Verification items for the finished model (mm, model axes). A direction names the side the tool comes from. Round coordinates to 2 decimals unless told otherwise and drop trailing zeros. Order: outer loops, then holes, each group sorted by start corner. A loop starts at its lowest first (then second) coordinate and runs counter-clockwise, first axis right, second up. Notation, with made-up numbers: M -17,68 L 33,68 A30 cw 33,107 Z; hole C 56.5,75 d5. An arc over 180 degrees is marked long. Answer as a JSON object with one key per item and string values. Group by question number.
```python
from build123d import *

# Parameters (mm, degrees)
IZIM1_R                                           = 52.5
IZIM1_R_2                                         = 21
Y_KSEKLIK_EKSTR_ZYON1_DEPTH                       = 10
Y_KSEKLIK_EKSTR_ZYON1_DRAFT                       = 4.33
M8_ALT_GEN_ALYAN_BA_L_K_R_VIDA_IN_HAV_D           = 9
M8_ALT_GEN_ALYAN_BA_L_K_R_VIDA_IN_HAV_DEPTH       = 22.25
M8_ALT_GEN_ALYAN_BA_L_K_R_VIDA_IN_HAV_CBORE_D     = 15
M8_ALT_GEN_ALYAN_BA_L_K_R_VIDA_IN_HAV_CBORE_DEPTH = 8.6
M8_ALT_GEN_ALYAN_BA_L_K_R_VIDA_IN_HAV_TIP         = 2.703872786
IZIM4_R                                           = 22
IZIM4_R_2                                         = 21
Y_KSEKLIK_EKSTR_ZYON2_DEPTH                       = 10


with BuildPart() as part:
    # Çizim1 → Yükseklik-Ekstrüzyon1 (with draft: the straight prism first)
    with BuildSketch(Plane.XY):
        Circle(IZIM1_R)
        Circle(IZIM1_R_2, mode=Mode.SUBTRACT)
    extrude(amount=Y_KSEKLIK_EKSTR_ZYON1_DEPTH)
    # Yükseklik-Ekstrüzyon1: the draft: its side faces are tilted about the plane it starts from
    y_kseklik_ekstr_zyon1_sides = [part.faces().sort_by_distance(p)[0] for p in [
        (-52.5, 0, 5),
        (-21, 0, 5),
    ]]
    draft(y_kseklik_ekstr_zyon1_sides, Plane.XY, Y_KSEKLIK_EKSTR_ZYON1_DRAFT)

    # M8 Altıgen Alyan Başlı Kör Vida İçin Havşa1
    with Locations(Plane.XY.offset(10)):
        with Locations((14.701198769, 35.58264682), (-35.58264682, 14.701198769), (-14.701198769, -35.58264682), (35.58264682, -14.701198769)):
            CounterBoreHole(M8_ALT_GEN_ALYAN_BA_L_K_R_VIDA_IN_HAV_D / 2, M8_ALT_GEN_ALYAN_BA_L_K_R_VIDA_IN_HAV_CBORE_D / 2, M8_ALT_GEN_ALYAN_BA_L_K_R_VIDA_IN_HAV_CBORE_DEPTH, depth=M8_ALT_GEN_ALYAN_BA_L_K_R_VIDA_IN_HAV_DEPTH)
            with Locations((0, 0, -(M8_ALT_GEN_ALYAN_BA_L_K_R_VIDA_IN_HAV_DEPTH + M8_ALT_GEN_ALYAN_BA_L_K_R_VIDA_IN_HAV_TIP / 2))):  # 118° drill point
                Cone(0, M8_ALT_GEN_ALYAN_BA_L_K_R_VIDA_IN_HAV_D / 2, M8_ALT_GEN_ALYAN_BA_L_K_R_VIDA_IN_HAV_TIP, mode=Mode.SUBTRACT)

    # Çizim4 → Yükseklik-Ekstrüzyon2 (add)
    with BuildSketch(Plane.XY):
        Circle(IZIM4_R)
        Circle(IZIM4_R_2, mode=Mode.SUBTRACT)
    extrude(amount=Y_KSEKLIK_EKSTR_ZYON2_DEPTH)


solid = part.part
```
Q1. Release check for a two-part mould opening along X. For faces 3 (the face through (22, 1, 10)), 4 (the face through (-39.875, 16.053, 0.69)), 5 (the face through (49.399, 15.556, 9.374)), 6 (the face through (-11, -39, 1.4)) record: released by +X, released by -X, zero draft, split by the parting line, or undercut.
Q2. Tool access check on faces 1 (the face through (-1, -23, 0)), 2 (the face through (-16.327, -42.904, 5.76)). Record the directions out of +Z, -Z, +X, -X, +Y, -Y that give a thin tool (end or side, any length) a straight path to the whole face; none if there is none.
Q3. Thickness scan on line 1 (X direction, y = 17, z = 5.5); line 2 (Y direction, x = 8.5, z = 8.75); line 3 (Y direction, x = 18, z = 1). Record the ranges inside material, lowest first. Write a range as from..to.
Q4. Cross-section at D-D, the plane z = 3. Record the cut outline in (x, y), then the cut area to 3 significant figures.
Q5. Gauge pin test, flat ends, axial feed: pin 1 Ø3 at (x, z) = (33.5, 3) entering from +Y; pin 2 Ø5 at (x, z) = (-38, 6.5) entering from +Y; pin 3 Ø4.5 at (x, y) = (38.5, -15) entering from +Z. Record the tip position at first contact, or that the pin passes through.
Q6. Cross-section at C-C, the plane z = 8.75. Record the cut outline in (x, y).
Q7. Cross-section at A-A, the plane y = 0. Record the cut outline in (x, z), then the cut area to 3 significant figures.
Conclusion:
{
 "1": {"face 3": "zero draft", "face 4": "undercut", "face 5": "split by the parting line", "face 6": "undercut"},
 "2": {"face 1": "-Z, +X, -X, +Y, -Y", "face 2": "+Z"},
 "3": {"line 1": "-49.23..-42.72, -28.44..-12.33, 12.33..49.23", "line 2": "-51.14..-19.2, 19.2..31.36, 39.8..51.14", "line 3": "-49.24..-10.82, 10.82..32.52, 38.64..49.24"},
 "4": {"outline": "C 0,0 d104.55; hole C -35.58,14.7 d15; hole C -14.7,-35.58 d15; hole C 0,0 d42; hole C 14.7,35.58 d15; hole C 35.58,-14.7 d15", "area": "6,490 mm2"},
 "5": {"pin 1": "y = 41.34", "pin 2": "y = 38.02", "pin 3": "z = 1.4"},
 "6": {"outline": "C 0,0 d103.67; hole C -35.58,14.7 d15; hole C -14.7,-35.58 d15; hole C 0,0 d42; hole C 14.7,35.58 d15; hole C 35.58,-14.7 d15"},
 "7": {"outline": "M -52.5,0 L -21,0 L -21,10 L -51.74,10 Z; M 21,0 L 52.5,0 L 51.74,10 L 21,10 Z", "area": "622 mm2"}
}
